Design review of the part built by this model. Coordinates are the model's own, in mm. Face numbers are marked on the shaded views. A direction names the side the tool comes from. Coordinates: 2 decimals unless noted, no trailing zeros. Loops run counter-clockwise (first coordinate to the right, second up) from the corner with the lowest first, then second, coordinate; pieces in that order, holes last.
Q1. Add section C-C on z = 0. Give the boundary of the cut face in (x, y), and give its area (3 significant figures).
Q2. Draft analysis for pull direction X (two halves, no side actions). For the marked faces 1, 2 and 3, state which applies: released by +X, released by -X, zero draft, split by the parting line, or undercut.
Q3. For P1, Ø1.4, axis at x = 0, z = 0, coming from the +Y side; P2, Ø2, axis at y = 15.5, z = 2.5, coming from the -X side; P3, Ø4, axis at x = 3.5, y = 19, coming from the +Z side; P4, Ø1.2, axis at x = 6, z = 0, coming from the -Y side, all flat-tipped, find the tip position at first contact; note any pin that passes through.
Q4. Add section D-D on x = -6.5. Give the boundary of the cut face in (y, z), and give its area (3 significant figures).
Q5. Machinability: for the marked faces 4, 5, 6 and 7, which of the approach directions +Z, -Z, +X, -X, +Y, -Y give a long, thin tool a straight path to every point of the face, cutting with its end or side? Answer none if there is none.
Q6. Wall thickness on probe 1 along X at (y, z) = (31, 0); probe 2 along X at (y, z) = (18, -1.5); probe 3 along Y at (x, z) = (0, 0): over which ranges is each line inside the solid? List them lowest first.
Q7. Add section B-B on x = 0. Give the boundary of the cut face in (y, z), and give its area (3 significant figures).
Q8. Add section A-A on y = 26.5. Give the boundary of the cut face in (x, z).
Autodesk Inventor part; units mm, degrees
ref_plane "YZ Plane" through (0, 0, 0) normal (1, 0, 0) x (0, 1, 0)
ref_plane "XZ Plane" through (0, 0, 0) normal (0, 1, 0) x (-1, 0, 0)
ref_plane "XY Plane" through (0, 0, 0) normal (0, 0, 1) x (1, 0, 0)
sketch "Sketch1" plane through (0, 0, 0) normal (0, 1, 0) x (-1, 0, 0)
  circle A0 centre (0, 0) radius 8
  dimension "d0" = 16
extrude "Extrusion1" add sketch "Sketch1" along normal blind 3
sketch "Sketch2" plane through (0, 3, 0) normal (0, 1, 0) x (1, 0, 0)
  circle A0 centre (-6, 0) radius 1
  point P0 (0, 0)
  dimension "d3" = 2
  dimension "d4" = 6
extrude "Extrusion2" cut sketch "Sketch2" against normal blind 3
pattern_circular "Circular Pattern1" count 4 over 360 about axis through (0, -10, 0) along (0, 1, 0) of "Extrusion2"
sketch "Sketch3" plane through (0, 3, 0) normal (0, 1, 0) x (1, 0, 0)
  line L0 (3.9, 3.9) -> (-3.9, 3.9)
  line L1 (-3.9, 3.9) -> (-3.9, -3.9)
  line L2 (-3.9, -3.9) -> (3.9, -3.9)
  line L3 (3.9, -3.9) -> (3.9, 3.9)
  line L4 (3.9, 3.9) -> (-3.9, -3.9) construction
  line L5 (-3.9, 3.9) -> (3.9, -3.9) construction
  line L6 (-3.9, -3.9) -> (-1.9, -3.9)
  line L7 (-1.9, -3.9) -> (-1.9, -1.9)
  line L8 (-1.9, -1.9) -> (-3.9, -1.9)
  line L9 (-3.9, -1.9) -> (-3.9, -3.9)
  line L10 (-3.9, 3.9) -> (-1.9, 3.9)
  line L11 (-1.9, 3.9) -> (-1.9, 1.9)
  line L12 (-1.9, 1.9) -> (-3.9, 1.9)
  line L13 (-3.9, 1.9) -> (-3.9, 3.9)
  line L14 (3.9, -3.9) -> (1.9, -3.9)
  line L15 (1.9, -3.9) -> (1.9, -1.9)
  line L16 (1.9, -1.9) -> (3.9, -1.9)
  line L17 (3.9, -1.9) -> (3.9, -3.9)
  line L18 (3.9, 3.9) -> (1.9, 3.9)
  line L19 (1.9, 3.9) -> (1.9, 1.9)
  line L20 (1.9, 1.9) -> (3.9, 1.9)
  line L21 (3.9, 1.9) -> (3.9, 3.9)
  point P0 (0, 0)
  point P1 (3.9, 1.9)
  point P2 (1.9, 3.9)
  point P3 (-1.9, 3.9)
  point P4 (-1.9, -3.9)
  point P5 (1.9, -3.9)
  dimension "d10" = 7.8
  dimension "d11" = 7.8
  dimension "d14" = 2
  dimension "d15" = 2
extrude "Extrusion3" add sketch "Sketch3" along normal blind 31 contours L19 L20 L3 L16 L15 L2 L7 L8 L1 L12 L11 L0
sketch "Sketch4" plane through (0, 34, 0) normal (0, 1, 0) x (1, 0, 0)
  circle A0 centre (0, 0) radius 0.75
  dimension "d16" = 1.5
extrude "Extrusion4" cut sketch "Sketch4" against normal blind 8
properties part number "XC330_motor_adaptor"
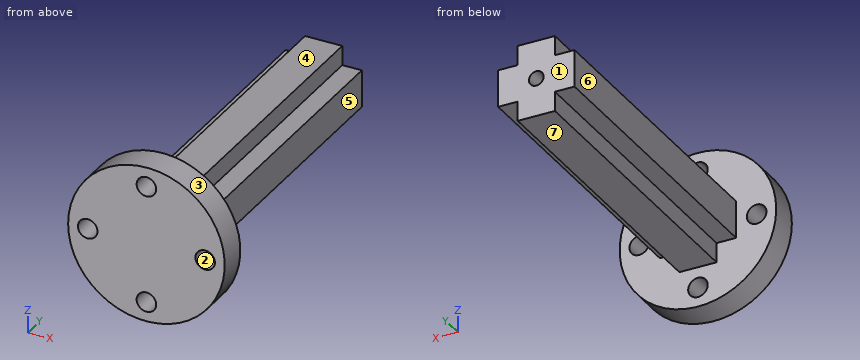
Entries:
1. outline: (-8, 0) - (-7, 0) - (-7, 3) - (-8, 3) - close; (-5, 0) - (5, 0) - (5, 3) - (3.9, 3) - (3.9, 34) - (0.75, 34) - (0.75, 26) - (-0.75, 26) - (-0.75, 34) - (-3.9, 34) - (-3.9, 3) - (-5, 3) - close; (7, 0) - (8, 0) - (8, 3) - (7, 3) - close
1. area: 266 mm2
2. face 1: zero draft
2. face 2: undercut
2. face 3: split by the parting line
3. P1: stops at y = 26
3. P2: stops at x = -3.9
3. P3: stops at z = 3.9
3. P4: passes through
4. outline: (0, -4.66) - (3, -4.66) - (3, -0.87) - (0, -0.87) - close; (0, 0.87) - (3, 0.87) - (3, 4.66) - (0, 4.66) - close
4. area: 22.8 mm2
5. face 4: +Z, +X, -X, +Y
5. face 5: +Z, -Z, +X, +Y
5. face 6: +Z, -Z, -X, +Y
5. face 7: -Z, +X, -X, +Y
6. probe 1: x = -3.9 to -0.75, 0.75 to 3.9
6. probe 2: x = -3.9 to 3.9
6. probe 3: y = 0 to 26
7. outline: (0, -8) - (3, -8) - (3, -7) - (0, -7) - close; (0, -5) - (3, -5) - (3, -3.9) - (34, -3.9) - (34, -0.75) - (26, -0.75) - (26, 0.75) - (34, 0.75) - (34, 3.9) - (3, 3.9) - (3, 5) - (0, 5) - close; (0, 7) - (3, 7) - (3, 8) - (0, 8) - close
7. area: 266 mm2
8. outline: (-3.9, -1.9) - (-1.9, -1.9) - (-1.9, -3.9) - (1.9, -3.9) - (1.9, -1.9) - (3.9, -1.9) - (3.9, 1.9) - (1.9, 1.9) - (1.9, 3.9) - (-1.9, 3.9) - (-1.9, 1.9) - (-3.9, 1.9) - close; hole circle Ø1.5 at (0, 0)
